```python
from build123d import *

# Parameters (mm, degrees)
SKETCH1_R                  = 25
BOSS_EXTRUDE1_DEPTH        = 33
CUT_EXTRUDE1_DEPTH         = 49.363209157
CUT_EXTRUDE1_DEPTH_BACK    = 49.363209157
SKETCH2_R                  = 12.5
BOSS_EXTRUDE2_START        = -28
BOSS_EXTRUDE2_DEPTH        = 5
BOSS_EXTRUDE2_DRAFT        = -10
BOSS_EXTRUDE3_START        = -16
BOSS_EXTRUDE3_DEPTH        = 12
BOSS_EXTRUDE5_START        = 28
BOSS_EXTRUDE5_DEPTH        = 5
BOSS_EXTRUDE5_TAPER        = 10
BOSS_EXTRUDE6_START        = 28
BOSS_EXTRUDE6_DEPTH        = 12
BOSS_EXTRUDE7_DEPTH        = 28
F_12_0_12_DIAMETER_HOLE1_D = 12
CIRPATTERN1_COUNT          = 4
CIRPATTERN1_ANGLE          = 90
CUT_EXTRUDE3_DEPTH         = 140.247980237
CUT_EXTRUDE3_DEPTH_BACK    = 56
FILLET1_R                  = 6


with BuildPart() as part:
    # Sketch1 → Boss-Extrude1 (new, symmetric)
    with BuildSketch(Plane.XY):
        Circle(SKETCH1_R)
    extrude(amount=BOSS_EXTRUDE1_DEPTH, both=True)

    # Sketch2 → Cut-Extrude1 (cut, two sides: drawn at the far end of the back side and taken through both)
    with BuildSketch(Plane.XY.offset(-CUT_EXTRUDE1_DEPTH_BACK)):
        Circle(SKETCH2_R)
    extrude(amount=CUT_EXTRUDE1_DEPTH + CUT_EXTRUDE1_DEPTH_BACK, mode=Mode.SUBTRACT)



with BuildPart() as body_2:
    # Sketch4 → Boss-Extrude2 (with draft: the straight prism first)
    with BuildSketch(Plane.XY.offset(BOSS_EXTRUDE2_START)):
        with BuildLine():
            ThreePointArc((90, 0), (63.639610307, 63.639610307), (0, 90))
            ThreePointArc((0, 90), (-15, 75), (0, 60))
            ThreePointArc((0, 60), (42.426406871, 42.426406871), (60, 0))
            ThreePointArc((60, 0), (75, -15), (90, 0))
        make_face()
    extrude(amount=-BOSS_EXTRUDE2_DEPTH)
    # Boss-Extrude2: the draft: its side faces are tilted about the plane it starts from
    boss_extrude2_sides = [body_2.faces().sort_by_distance(p)[0] for p in [
        (42.426406871, 42.426406871, -30.5),
        (75, -15, -30.5),
        (63.639610307, 63.639610307, -30.5),
        (-15, 75, -30.5),
    ]]
    draft(boss_extrude2_sides, Plane.XY.offset(BOSS_EXTRUDE2_START), BOSS_EXTRUDE2_DRAFT)


with BuildPart() as part_1:
    add(part.part)

    add(body_2.part)  # Boss-Extrude3 merges body 2
    # Sketch4<3> → Boss-Extrude3 (add)
    with BuildSketch(Plane.XY.offset(BOSS_EXTRUDE3_START)):
        with BuildLine():
            Line((15, 20), (15, 58.094750193))
            ThreePointArc((15, 58.094750193), (47.434164903, 36.742346142), (60, 0))
            ThreePointArc((60, 0), (75, -15), (90, 0))
            ThreePointArc((90, 0), (63.639610307, 63.639610307), (0, 90))
            ThreePointArc((0, 90), (-10.606601718, 85.606601718), (-15, 75))
            Line((-15, 75), (-15, 20))
            ThreePointArc((-15, 20), (0, 25), (15, 20))
        make_face()
    extrude(amount=-BOSS_EXTRUDE3_DEPTH)



with BuildPart() as body_2_2:
    # Sketch4<5> → Boss-Extrude5 (new body)
    with BuildSketch(Plane.XY.offset(BOSS_EXTRUDE5_START)):
        with BuildLine():
            ThreePointArc((90, 0), (63.639610307, 63.639610307), (0, 90))
            ThreePointArc((0, 90), (-15, 75), (0, 60))
            ThreePointArc((0, 60), (42.426406871, 42.426406871), (60, 0))
            ThreePointArc((60, 0), (75, -15), (90, 0))
        make_face()
    extrude(amount=BOSS_EXTRUDE5_DEPTH, taper=BOSS_EXTRUDE5_TAPER)


with BuildPart() as part_2:
    add(part_1.part)

    add(body_2_2.part)  # Boss-Extrude6 merges body 2 2
    # Sketch4<8> → Boss-Extrude6 (add)
    with BuildSketch(Plane.XY.offset(BOSS_EXTRUDE6_START)):
        with BuildLine():
            ThreePointArc((90, 0), (63.639610307, 63.639610307), (0, 90))
            ThreePointArc((0, 90), (-15, 75), (0, 60))
            ThreePointArc((0, 60), (42.426406871, 42.426406871), (60, 0))
            ThreePointArc((60, 0), (75, -15), (90, 0))
        make_face()
        with BuildLine():
            ThreePointArc((0, 60), (-10.606601718, 64.393398282), (-15, 75))
            Line((-15, 75), (-15, 20))
            ThreePointArc((-15, 20), (0, 25), (15, 20))
            Line((15, 20), (15, 58.094750193))
            ThreePointArc((15, 58.094750193), (7.560257549, 59.521781776), (0, 60))
        make_face()
    extrude(amount=-BOSS_EXTRUDE6_DEPTH)

    # Sketch10 → Boss-Extrude7 (add, symmetric)
    with BuildSketch(Plane.XY):
        with BuildLine():
            Line((-22.449944321, -11), (-75, -11))
            Line((-75, -11), (-75, -27))
            Line((-75, -27), (90, -27))
            Line((90, -27), (90, 0))
            Line((90, 0), (25, 0))
            ThreePointArc((25, 0), (5.645856533, -24.354143467), (-22.449944321, -11))
        make_face()
    extrude(amount=BOSS_EXTRUDE7_DEPTH, both=True)

    # Ø12.0 (12) Diameter Hole1 (through all)
    with Locations(Plane.XY.offset(33)):
        with Locations((0, 75)):
            f_12_0_12_diameter_hole1 = Hole(F_12_0_12_DIAMETER_HOLE1_D / 2)

    # CirPattern1: Ø12.0 (12) Diameter Hole1 ×4 about axis
    cirpattern1_axis = Axis((0, 0, 0), (0, 0, -1))
    for i in range(1, CIRPATTERN1_COUNT):
        add(f_12_0_12_diameter_hole1.rotate(cirpattern1_axis, i * CIRPATTERN1_ANGLE / (CIRPATTERN1_COUNT - 1)), mode=Mode.SUBTRACT)

    # Sketch11 → Cut-Extrude3 (cut, two sides: drawn at the far end of the back side and taken through both)
    with BuildSketch(Plane(origin=(0, -11, 0), x_dir=(1, 0, 0), z_dir=(0, 1, 0)).offset(-CUT_EXTRUDE3_DEPTH_BACK)):
        with BuildLine():
            Line((-55, 10), (-75, 10))
            Line((-75, 10), (-75, -10))
            Line((-75, -10), (-55, -10))
            ThreePointArc((-55, -10), (-45, 0), (-55, 10))
        make_face()
    extrude(amount=CUT_EXTRUDE3_DEPTH + CUT_EXTRUDE3_DEPTH_BACK, mode=Mode.SUBTRACT)

    # Fillet1
    # the kernel refuses this fillet: 6 mm, written as the material it adds along each edge
    with BuildSketch(Plane(origin=(60, 0, -16), x_dir=(-0.055641755903696445, 0.9984507974857616, 0), z_dir=(0, 0, -1))) as fillet1_piece_1:
        with BuildLine():
            CenterArc((6.343160173, -5.990704785), FILLET1_R, 86.810314896, 96.379370208)
            Line((0.352455388, -6.32455532), (0, 0))
            ThreePointArc((0, 0), (3.338505354, 0.092952151), (6.677010708, 0))
        make_face()
    extrude(amount=12)
    with BuildSketch(Plane(origin=(60, 0, 28), x_dir=(-1, 0, 0), z_dir=(0, 0, -1))) as fillet1_piece_2:
        with BuildLine():
            CenterArc((6.33436854, 6), FILLET1_R, 173.620629792, 96.379370208)
            ThreePointArc((0.3715206, 6.666666667), (0.092952151, 3.338505354), (0, 0))
            Line((0, 0), (6.33436854, 0))
        make_face()
    extrude(amount=12)
    with BuildSketch(Plane(origin=(25, 0, 28), x_dir=(-0.09723494563874313, 0.9952614557726179, 0), z_dir=(0, 0, -1))) as fillet1_piece_3:
        with BuildLine():
            CenterArc((5.445156956, 5.971568735), FILLET1_R, 185.579968436, 78.840063128)
            Line((-0.526411779, 5.388159061), (0, 0))
            ThreePointArc((0, 0), (2.430873641, 0.118463606), (4.861747282, 0))
        make_face()
    extrude(amount=56)
    with BuildSketch(Plane(origin=(-22.449944321, -11, 28), x_dir=(-0.30391401052504813, 0.9526994668868987, 0), z_dir=(0, 0, -1))) as fillet1_piece_4:
        with BuildLine():
            CenterArc((8.191325007, -5.935464984), FILLET1_R, 98.411041025, 99.281799087)
            Line((2.475128206, -7.758949048), (0, 0))
            ThreePointArc((0, 0), (3.656841521, -0.268895898), (7.313683042, 0))
        make_face()
    extrude(amount=56)


solid = part_2.part
```
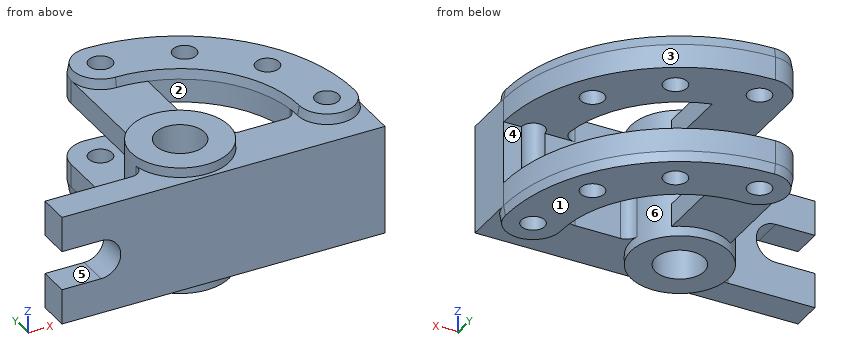
Verification items for the finished model (mm, model axes). Face numbers are marked on the shaded views. A direction names the side the tool comes from. Give positions to 0.01 mm unless a question says otherwise; leave off trailing zeros. Order: outer loops, then holes, each group sorted by start corner. A loop starts at its lowest first (then second) coordinate and runs counter-clockwise, first axis right, second up. Notation, with made-up numbers: (-4.75, -17.75) -> (3.25, -17.75) arc R23 ccw to (3.25, -6.75) -> close; hole circle Ø1 at (34, 67.25). An arc over 180 degrees is marked (long way). Use a Markdown table: item, result.
1) Section check B-B, the plane y = -18. Record the boundary of the cut face in (x, z).
Results:
| item | result |
|---|---|
| outline | (-75, -28) -> (-17.35, -28) -> (-17.35, -33) -> (17.35, -33) -> (17.35, -28) -> (90, -28) -> (90, 28) -> (17.35, 28) -> (17.35, 33) -> (-17.35, 33) -> (-17.35, 28) -> (-75, 28) -> (-75, 10) -> (-55, 10) arc R10 cw to (-55, -10) -> (-75, -10) -> close |
2) Tool access check on the marked faces 4, 5 and 6. Record the directions out of +Z, -Z, +X, -X, +Y, -Y that give a thin tool (end or side, any length) a straight path to the whole face; none if there is none.
Results:
| item | result |
|---|---|
| face 4 | +X, +Y |
| face 5 | -X, +Y, -Y |
| face 6 | none |
3) Section check D-D, the plane z = -18.5. Record the boundary of the cut face in (x, y).
Results:
| item | result |
|---|---|
| outline | (-75, -27) -> (90, -27) -> (90, 0) arc R90 ccw to (0, 90) arc R15 ccw to (-15, 75) -> (-15, 20) arc R25 ccw to (-24.67, -4.03) arc R6 cw to (-30.59, -11) -> (-75, -11) -> close; hole circle Ø25 at (0, 0); hole circle Ø12 at (0, 75); hole (15, 20) arc R25 cw to (24.53, 4.84) arc R6 ccw to (30.41, 0) -> (53.67, 0) arc R6 ccw to (59.63, 6.67) arc R60 ccw to (15, 58.09) -> close; hole circle Ø12 at (37.5, 64.95); hole circle Ø12 at (64.95, 37.5); hole circle Ø12 at (75, 0) |
4) Section check C-C, the plane x = -37.5. Record the boundary of the cut face in (y, z).
Results:
| item | result |
|---|---|
| outline | (-27, -28) -> (-11, -28) -> (-11, 28) -> (-27, 28) -> close |
5) Depth check by flat-ended pin: pin 1 Ø10 at (y, z) = (62, -6.5) entering from -X; pin 2 Ø9.5 at (y, z) = (38.5, -20) entering from +X; pin 3 Ø13 at (y, z) = (55, 24) entering from -X; pin 4 Ø8 at (x, y) = (48.5, -10.5) entering from +Z. Enter the tip coordinate at first touch or a pass-through.
Results:
| item | result |
|---|---|
| pin 1 | through |
| pin 2 | x = 83.43 |
| pin 3 | x = -15 |
| pin 4 | z = 28 |
6) Mould release check, pull along X, two halves, no side actions. Record for the marked faces 1, 2 and 3: pulls with the +X half, pulls with the -X half, needs draft (parallel to the pull), parting line crosses it, or undercut.
Results:
| item | result |
|---|---|
| face 1 | needs draft |
| face 2 | undercut |
| face 3 | pulls with the +X half |
7) Material ranges on probe 1 along Z at (x, y) = (-9, 50); probe 2 along Z at (x, y) = (51, 61); probe 3 along Y at (x, z) = (42, -18), recorded low to high.
Results:
| item | result |
|---|---|
| probe 1 | -28 to -16, 16 to 28 |
| probe 2 | -33 to -16, 16 to 33 |
| probe 3 | -27 to 0, 42.85 to 60.98, 68.92 to 79.6 |
8) Section check A-A, the plane z = 0. Record the boundary of the cut face in (x, y).
Results:
| item | result |
|---|---|
| outline | (-45, -27) -> (90, -27) -> (90, 0) -> (81, 0) arc R6 cw to (69, 0) -> (30.41, 0) arc R6 cw to (24.53, 4.84) arc R25 ccw to (-24.67, -4.03) arc R6 cw to (-30.59, -11) -> (-45, -11) -> close; hole circle Ø25 at (0, 0) |
